Job drawing, mm, ordinate dimensions from the low corner. One solid piece. Give positions to 0.01 mm unless a question says otherwise; leave off trailing zeros. Order: outer loops, then holes, each group sorted by start corner. A loop starts at its lowest first (then second) coordinate and runs counter-clockwise, first axis right, second up. Notation, with made-up numbers: M 46.25,74.25 L 95.25,74.25 A13 ccw 95.25,94.25 Z; hole C 50,-25.5 d9. An arc over 180 degrees is marked long. Put each result on its own line as item: value. Start each with the question number.
1) Cut at C-C (y = 1.75). Give the number of separate pieces and of enclosed holes in the cut face, and give its area (3 significant figures).
2) Cut at D-D (z = 28). Write the cut outline in (x, y).
3) Pin check, flat tips, straight feed: pin 1 (1.5 mm diameter, centred on x = 34, y = 1, fed in from +Z) (1 decimal); pin 2 (1.5 mm diameter, centred on x = 41.5, y = 2, fed in from +Z); pin 3 (0.9 mm diameter, centred on x = 36.5, y = 1.5, fed in from -Z). Stop position of each tip, or through.
4) Cut at B-B (z = 40). Write the cut outline in (x, y), and give its area (3 significant figures).
5) Drill centre lines: line 1 (X direction, y = 1.05, z = 20); line 2 (Z direction, x = 39.5, y = 2.7) (1 decimal); line 3 (X direction, y = 1.7, z = 40). Where is each one in solid material? Low to high. Write a range as [from, to].
6) Cut at A-A (x = 13). Write the cut outline in (y, z), and give its area (3 significant figures).
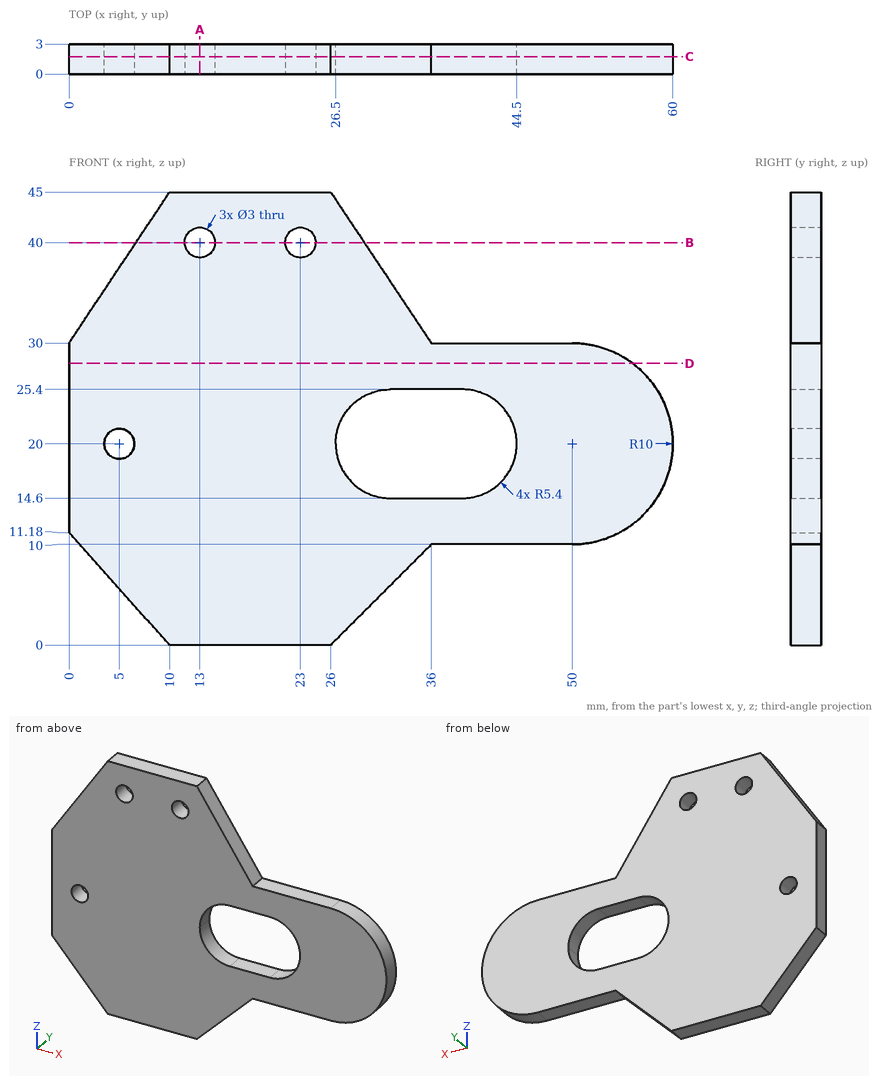
Solution:
1. separate pieces: 1
1. enclosed holes: 4
1. area: 1,610 mm²
2. outline: M 0,0 L 56,0 L 56,3 L 0,3 Z
3. pin 1: z = 34.1
3. pin 2: z = 30
3. pin 3: z = 10
4. outline: M 6.67,0 L 11.5,0 L 11.5,3 L 6.67,3 Z; M 14.5,0 L 21.5,0 L 21.5,3 L 14.5,3 Z; M 24.5,0 L 29.33,0 L 29.33,3 L 24.5,3 Z
4. area: 50.0 mm²
5. line 1: [0, 3.5], [6.5, 26.5], [44.5, 60]
5. line 2: [10, 14.6], [25.4, 30]
5. line 3: [6.67, 11.5], [14.5, 21.5], [24.5, 29.33]
6. outline: M 0,0 L 3,0 L 3,38.5 L 0,38.5 Z; M 0,41.5 L 3,41.5 L 3,45 L 0,45 Z
6. area: 126 mm²
